Part model, mm, in its own coordinate system. Face numbers are marked on the shaded views. A direction names the side the tool comes from. Give positions to 0.01 mm unless a question says otherwise; leave off trailing zeros. Write each loop counter-clockwise with the first axis right and the second up, starting at its lowest first coordinate (ties: lowest second). Pieces come first, ordered by that corner, then holes. Notation, with made-up numbers: (36.25, -13) - (70.25, -13) arc R26 ccw to (70.25, 7) - close; hole circle Ø1 at (3.5, 0). An arc over 180 degrees is marked (long way). Answer as a JSON object with one key per item and string values. Group by question number.
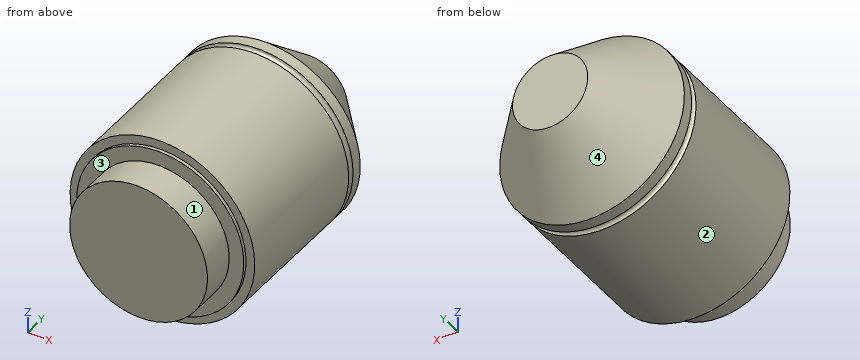
Autodesk Inventor part; units mm, degrees
ref_plane "YZ Plane" through (0, 0, 0) normal (1, 0, 0) x (0, 1, 0)
ref_plane "XZ Plane" through (0, 0, 0) normal (0, 1, 0) x (-1, 0, 0)
ref_plane "XY Plane" through (0, 0, 0) normal (0, 0, 1) x (1, 0, 0)
sketch "Skizze1" plane through (0, 0, 0) normal (1, 0, 0) x (0, 1, 0)
  line L0 (0, 13.5) -> (24, 13.5)
  line L1 (24, 13.5) -> (33.534, 5.5)
  line L2 (33.534, 5.5) -> (33.534, 0)
  line L3 (33.534, 0) -> (0, 0)
  line L4 (0, 0) -> (0, 13.5)
  arc A0 (21.35, 13.5) -> (22.35, 13.5) centre (21.85, 13.5) ccw
  line L5 (0, 0) -> (-0.5, 0)
  line L6 (-0.5, 0) -> (-0.5, 12.225)
  line L7 (-0.5, 12.225) -> (0, 12.225)
  line L8 (0, 12.225) -> (0, 0)
  line L9 (-0.5, 0) -> (-5.43, 0)
  line L10 (-5.43, 0) -> (-5.43, 10.08)
  line L11 (-5.43, 10.08) -> (-0.5, 10.08)
  line L12 (-0.5, 10.08) -> (-0.5, 0)
  point P0 (-0.5, 10.08)
  dimension "d0" = 24
  dimension "d1" = 140
  dimension "d2" = 5.5
  dimension "d3" = 1
  dimension "d4" = 0.5
  dimension "d5" = 1.65
  dimension "d6" = 0.5
  dimension "d7" = 12.225
  dimension "d8" = 4.93
  dimension "d9" = 10.08
revolve "Umdrehung1" add sketch "Skizze1" angle 360 about axis through (0, 33.534, 0) along (0, -1, 0) contours L0 A0 L1 L2 L3 L4 | L4 L5 L6 L7 | L9 L10 L11 L6
properties part number "00_10x_Objective_ViewSolutions_bm05073332"
1) Drop flat-ended pins along their axis: P1, Ø5, axis at y = 28, z = -8, coming from the -X side; P2, Ø3, axis at x = -5, z = -10.5, coming from the +Y side; P3, Ø4, axis at x = 9.5, z = -5, coming from the +Y side. Give the stop position or say it passes through.
2) Band-saw the part on D-D (y = 24.5). List the corners of the cut face in (x, z), plus the area to 3 significant figures.
3) Band-saw the part on A-A (x = 0). List the corners of the cut face in (y, z) (3 decimals), plus the area to 3 significant figures.
4) Mould opens along Z. For the marked faces 3 and 4 say: pulls with the +Z half, pulls with the -Z half, needs draft (parallel to the pull), parting line crosses it, or undercut.
5) Band-saw the part on C-C (y = -1). List the corners of the cut face in (x, z).
6) Which spindle directions (+Z, -Z, +X, -X, +Y, -Y) get a long thin tool onto all of the face, cutting with end or side? Do the marked faces 1 and 2. Say none if no direction does.
7) Band-saw the part on B-B (z = 0). List the corners of the cut face in (x, y) (3 decimals), plus the area to 3 significant figures.
8) Probe line 1 (Z direction, x = -0.5, y = 9); line 2 (X direction, y = 3, z = 2.75); line 3 (X direction, y = 4.5, z = -11). List the from-to ranges inside material, lowest first.
Verdict:
{
 "1": {"P1": "x = -9.88", "P2": "y = 28.02", "P3": "y = 29.68"},
 "2": {"outline": "circle Ø26.16 at (0, 0)", "area": "538 mm2"},
 "3": {"outline": "(-5.43, -10.08) - (-0.5, -10.08) - (-0.5, -12.225) - (0, -12.225) - (0, -13.5) - (21.35, -13.5) arc R0.5 cw to (22.35, -13.5) - (24, -13.5) - (33.534, -5.5) - (33.534, 5.5) - (24, 13.5) - (22.35, 13.5) arc R0.5 cw to (21.35, 13.5) - (0, 13.5) - (0, 12.225) - (-0.5, 12.225) - (-0.5, 10.08) - (-5.43, 10.08) - close", "area": "940 mm2"},
 "4": {"face 3": "needs draft", "face 4": "parting line crosses it"},
 "5": {"outline": "circle Ø20.16 at (0, 0)"},
 "6": {"face 1": "-Y", "face 2": "+Y, -Y"},
 "7": {"outline": "(-13.5, 0) - (-12.225, 0) - (-12.225, -0.5) - (-10.08, -0.5) - (-10.08, -5.43) - (10.08, -5.43) - (10.08, -0.5) - (12.225, -0.5) - (12.225, 0) - (13.5, 0) - (13.5, 21.35) arc R0.5 cw to (13.5, 22.35) - (13.5, 24) - (5.5, 33.534) - (-5.5, 33.534) - (-13.5, 24) - (-13.5, 22.35) arc R0.5 cw to (-13.5, 21.35) - close", "area": "940 mm2"},
 "8": {"line 1": "-13.49 to 13.49", "line 2": "-13.22 to 13.22", "line 3": "-7.83 to 7.83"}
}
